Here's how the part is built. I have some questions about the finished solid (model axes, mm). Face numbers are marked on the shaded views. A direction names the side the tool comes from. Coordinates: 2 decimals unless noted, no trailing zeros. Write each loop counter-clockwise with the first axis right and the second up, starting at its lowest first coordinate (ties: lowest second). Pieces come first, ordered by that corner, then holes. Notation, with made-up numbers: (40, 56) - (54, 56) arc R12 ccw to (54, 79) - close; hole circle Ø2 at (9.5, -16.5). An arc over 180 degrees is marked (long way). Answer in a Markdown table with one row per item. Add a question column.
Item 1: We'd pull the mould along X, two halves only. Please class the marked faces 1, 2, 3 and 4: +X half, -X half, draft (parallel to the pull), parting line (faces both ways), or undercut.
Item 2: Imagine slicing it at A-A (x = 10.2). Please give me the cut outline in (y, z).
Item 3: Which directions (+Z, -Z, +X, -X, +Y, -Y) give clear straight access to the entire face, cutting with the end or side of a thin tool? Please do the marked faces 5 and 6.
Item 4: If I drill on probe 1 along Y at (x, z) = (10.2, -18.35); probe 2 along Y at (x, z) = (11.75, -19.5); probe 3 along Z at (x, y) = (10.25, 13.5), over which ranges is the centre line in solid material (lowest first)? Write a range as from..to.
Item 5: I'm going to push flat-ended pins straight in: pin 1 (4 mm diameter, centred on x = 9, z = -27, fed in from -Y); pin 2 (1 mm diameter, centred on x = 10.5, y = -6, fed in from +Z); pin 3 (4 mm diameter, centred on x = 7, y = -2.5, fed in from -Z). Where does each tip first touch, or does it pass through?
Item 6: Imagine slicing it at B-B (x = 13.5). Please give me the cut outline in (y, z), plus the area to 3 significant figures.
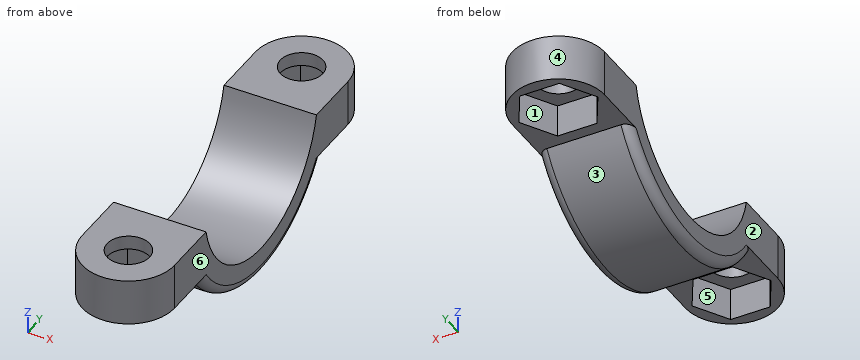
Autodesk Inventor part; units mm, degrees
ref_plane "YZ Plane" through (0, 0, 0) normal (1, 0, 0) x (0, 1, 0)
ref_plane "XZ Plane" through (0, 0, 0) normal (0, 1, 0) x (-1, 0, 0)
ref_plane "Arbeitsebene1" through (0, 0, -17.5) normal (0, 0, 1) x (1, 0, 0)
sketch "Skizze1" plane through (0, 0, -17.5) normal (0, 0, 1) x (1, 0, 0)
  arc A0 (5.2, -17) -> (15.2, -17) centre (10.2, -17) ccw
  circle A1 centre (10.2, -17) radius 2.3
  circle A2 centre (10.2, 17) radius 2.3
  arc A3 (15.2, 17) -> (5.2, 17) centre (10.2, 17) ccw
  line L0 (15.2, 17) -> (15.2, -17)
  line L1 (5.2, -17) -> (5.2, 17)
  point P0 (0, 0)
  dimension "d17" = 34
  dimension "d19" = 5
  dimension "d20" = 5
  dimension "d21" = 4.6
  dimension "d22" = 4.6
  dimension "d23" = 5.2
  dimension "d24" = 15.2
  dimension "d25" = 17
extrude "Extrusion1" add sketch "Skizze1" against normal blind 15
sketch "Skizze2" plane through (15.2, -17, -17.5) normal (1, 0, 0) x (0, 0, -1)
  circle A0 centre (-2.4, 17) radius 11.1
  circle A1 centre (-2.4, 17) radius 14.1
  line L0 (0, 39) -> (15, 39)
  line L1 (5, 39) -> (5, 29.0021)
  line L2 (5, 39) -> (-2.0976, 39.0148)
  line L3 (-2.0976, 39.0148) -> (-4.3191, 38.5001)
  line L4 (-4.3191, 38.5001) -> (-4.8354, 27.8295)
  line L5 (-4.8906, 6.183) -> (-12.1302, -16.582)
  line L6 (-12.1302, -16.582) -> (7.7221, -22.1422)
  line L7 (7.7221, -22.1422) -> (5, -5)
  line L8 (0, -5) -> (15, -5)
  line L9 (5, -5) -> (5, 4.9979)
  line L10 (0, 0) -> (0, -5)
  line L11 (36.0228, 70.8555) -> (-22.3921, 70.8555)
  line L12 (-22.3921, 70.8555) -> (-22.3921, -28.3632)
  line L13 (-22.3921, -28.3632) -> (36.0228, -28.3632)
  line L14 (36.0228, -28.3632) -> (36.0228, 70.8555)
  point P0 (-17.5, 17)
  point P1 (-5.8022, 3.3166)
  point P2 (-4.6862, 30.9134)
  dimension "d5" = 3
  dimension "d6" = 5
  dimension "d26" = 44
  dimension "d27" = 22
  dimension "d28" = 22.2
  dimension "d29" = 15.1
extrude "Extrusion2" cut sketch "Skizze2" against normal blind 10 contours A0 | L14 L13 L12 L11
sketch "Skizze3" plane through (15.2, -17, -22.5) normal (0, 0, -1) x (-1, 0, 0)
  circle A0 centre (5, 34) radius 2.3
  line L0 (2.8638, 30.3) -> (0.7276, 34)
  line L1 (0.7276, 34) -> (2.8638, 37.7)
  line L2 (2.8638, 37.7) -> (7.1362, 37.7)
  line L3 (7.1362, 37.7) -> (9.2724, 34)
  line L4 (9.2724, 34) -> (7.1362, 30.3)
  line L5 (7.1362, 30.3) -> (2.8638, 30.3)
  line L6 (0.7276, 0) -> (2.8638, 3.7)
  line L7 (2.8638, 3.7) -> (7.1362, 3.7)
  line L8 (7.1362, 3.7) -> (9.2724, 0)
  line L9 (9.2724, 0) -> (7.1362, -3.7)
  line L10 (7.1362, -3.7) -> (2.8638, -3.7)
  line L11 (2.8638, -3.7) -> (0.7276, 0)
  point P0 (15.2, 17)
  point P1 (5, 34)
  point P2 (5, 0)
  point P3 (5, 0)
  point P4 (5.6446, 34.7922)
  point P5 (4.3554, 34.7922)
  dimension "d9" = 7.4
  dimension "d10" = 7.4
extrude "Extrusion3" cut sketch "Skizze3" along normal blind 10 and the other way blind 3.5 contours A0 | L0 L1 L2 L3 L4 L5 | L6 L7 L8 L9 L10 L11
fillet "Rundung1" radius 1 2 edges at (15.2, 0, -29.2) (5.2, 0, -29.2)
equation "\"d20\" = d19"
equation "\"d27\" = 0.5 * d26"
equation "\"d10\" = d9"
properties part number "Bracket22_2"
Here are the results:
| question | item | result |
|---|---|---|
| 1 | face 1 | undercut |
| 1 | face 2 | -X half |
| 1 | face 3 | draft |
| 1 | face 4 | parting line |
| 2 | outline | (-22, -22.5) - (-20.7, -22.5) - (-20.7, -19) - (-19.3, -19) - (-19.3, -17.5) - (-22, -17.5) - close; (-14.7, -19) - (-13.3, -19) - (-13.3, -22.5) - (-12, -22.5) arc R14.1 ccw to (12, -22.5) - (13.3, -22.5) - (13.3, -19) - (14.7, -19) - (14.7, -17.5) - (10.84, -17.5) arc R11.1 cw to (-10.84, -17.5) - (-14.7, -17.5) - close; (19.3, -19) - (20.7, -19) - (20.7, -22.5) - (22, -22.5) - (22, -17.5) - (19.3, -17.5) - close |
| 3 | face 5 | -Z |
| 3 | face 6 | +Z, -Z, +X, +Y, -Y |
| 4 | probe 1 | y = -22..-19.3, -14.7..-10.61, 10.61..14.7, 19.3..22 |
| 4 | probe 2 | y = -21.75..-20.7, -13.3..-10.19, 10.19..13.3, 20.7..21.75 |
| 4 | probe 3 | z = -19..-17.5 |
| 5 | pin 1 | stops at y = -10.04 |
| 5 | pin 2 | stops at z = -24.1 |
| 5 | pin 3 | stops at z = -29.19 |
| 6 | outline | (-20.76, -22.5) - (-18.68, -22.5) - (-18.68, -19) - (-15.32, -19) - (-15.32, -22.5) - (-12, -22.5) arc R14.1 ccw to (12, -22.5) - (15.32, -22.5) - (15.32, -19) - (18.68, -19) - (18.68, -22.5) - (20.76, -22.5) - (20.76, -17.5) - (10.84, -17.5) arc R11.1 cw to (-10.84, -17.5) - (-20.76, -17.5) - close |
| 6 | area | 157 mm2 |
